Verification items for the finished model (mm, model axes). A direction names the side the tool comes from. Round coordinates to 2 decimals unless told otherwise and drop trailing zeros. Write each loop counter-clockwise with the first axis right and the second up, starting at its lowest first coordinate (ties: lowest second). Pieces come first, ordered by that corner, then holes. Notation, with made-up numbers: (-10, 3) - (25, 3) arc R20 cw to (25, 40) - close; hole circle Ø9 at (3.5, 35). An arc over 180 degrees is marked (long way). Answer as a JSON object with one key per item and string values.
```python
from build123d import *

# Parameters (mm, degrees)
SKIZZE1_W                       = 100
SKIZZE1_H                       = 66
AUFSATZ_LINEAR_AUSTRAGEN1_DEPTH = 1.5
SKIZZE2_W                       = 61
SKIZZE2_H                       = 14
AUFSATZ_LINEAR_AUSTRAGEN2_DEPTH = 14
SKIZZE6_W                       = 82.5
SKIZZE6_H                       = 14
AUFSATZ_LINEAR_AUSTRAGEN4_DEPTH = 4
SKIZZE3_R                       = 3
AUFSATZ_LINEAR_AUSTRAGEN3_DEPTH = 20
DURCHGANGSLOCH_F_R_M31_D        = 3.4
SKIZZE7_W                       = 35
SKIZZE7_H                       = 18
AUFSATZ_LINEAR_AUSTRAGEN5_DEPTH = 10


with BuildPart() as part:
    # Skizze1 → Aufsatz-Linear austragen1 (new body)
    with BuildSketch(Plane(origin=(0, 0, 0), x_dir=(1, 0, 0), z_dir=(0, 1, 0))):
        Rectangle(SKIZZE1_W, SKIZZE1_H)
    extrude(amount=AUFSATZ_LINEAR_AUSTRAGEN1_DEPTH)

    # Skizze2 → Aufsatz-Linear austragen2 (add)
    with BuildSketch(Plane(origin=(0, 1.5, 0), x_dir=(1, 0, 0), z_dir=(0, 1, 0))):
        with Locations((0.5, 21)):
            Rectangle(SKIZZE2_W, SKIZZE2_H)
    extrude(amount=AUFSATZ_LINEAR_AUSTRAGEN2_DEPTH)

    # Skizze6 → Aufsatz-Linear austragen4 (add)
    with BuildSketch(Plane(origin=(0, 1.5, 0), x_dir=(1, 0, 0), z_dir=(0, 1, 0))):
        with Locations((0.5, 21)):
            Rectangle(SKIZZE6_W, SKIZZE6_H)
    extrude(amount=AUFSATZ_LINEAR_AUSTRAGEN4_DEPTH)

    # Skizze3 → Aufsatz-Linear austragen3 (add)
    with BuildSketch(Plane(origin=(0, 1.5, 0), x_dir=(1, 0, 0), z_dir=(0, 1, 0))):
        with Locations((34, 1.5)):
            Circle(SKIZZE3_R)
    extrude(amount=AUFSATZ_LINEAR_AUSTRAGEN3_DEPTH)

    # Durchgangsloch für M31 (through all)
    with Locations(Plane(origin=(0, 1.5, 0), x_dir=(1, 0, 0), z_dir=(0, 1, 0))):
        with Locations((-46, -27.400776428), (-46, 27.400776428), (46, 27.400776428), (46, -27.400776428)):
            Hole(DURCHGANGSLOCH_F_R_M31_D / 2)

    # Skizze7 → Aufsatz-Linear austragen5 (add)
    with BuildSketch(Plane(origin=(0, 1.5, 0), x_dir=(1, 0, 0), z_dir=(0, 1, 0))):
        with Locations((-24.5, -0.5)):
            Rectangle(SKIZZE7_W, SKIZZE7_H)
    extrude(amount=AUFSATZ_LINEAR_AUSTRAGEN5_DEPTH)


solid = part.part
```
1. Material ranges on probe 1 along Z at (x, y) = (-46, 0.9); probe 2 along Z at (x, y) = (-20, 6); probe 3 along Y at (x, z) = (-39, 23), recorded low to high. Write a range as from..to.
Completed:
{"probe 1": "z = -33..-29.1, -25.7..25.7, 29.1..33", "probe 2": "z = -28..-14, -8.5..9.5", "probe 3": "y = 0..1.5"}
2. Go/stop test with flat-tipped pins: pin 1 (2 mm diameter, centred on x = 46, z = 27.4, fed in from +Y); pin 2 (10 mm diameter, centred on x = 14.5, z = -17, fed in from +Y); pin 3 (8.5 mm diameter, centred on x = 36.5, z = -21.5, fed in from +Y); pin 4 (1 mm diameter, centred on x = -5, y = 7, fed in from +Z). Record where each tip stops, or that it passes through.
Completed:
{"pin 1": "passes through", "pin 2": "stops at y = 15.5", "pin 3": "stops at y = 5.5", "pin 4": "stops at z = -14"}
3. Cross-section at B-B (y = 8.75). Record the boundary of the cut face in (x, z).
Completed:
{"outline": "(-42, -8.5) - (-7, -8.5) - (-7, 9.5) - (-42, 9.5) - close; (-30, -28) - (31, -28) - (31, -14) - (-30, -14) - close; circle Ø6 at (34, -1.5)"}
4. Cross-section at D-D (x = 15). Record the boundary of the cut face in (y, z).
Completed:
{"outline": "(0, -33) - (1.5, -33) - (1.5, -28) - (15.5, -28) - (15.5, -14) - (1.5, -14) - (1.5, 33) - (0, 33) - close"}
5. Cross-section at A-A (x = -46). Record the boundary of the cut face in (y, z), plus the area to 3 significant figures.
Completed:
{"outline": "(0, -33) - (1.5, -33) - (1.5, -29.1) - (0, -29.1) - close; (0, -25.7) - (1.5, -25.7) - (1.5, 25.7) - (0, 25.7) - close; (0, 29.1) - (1.5, 29.1) - (1.5, 33) - (0, 33) - close", "area": "88.8 mm^2"}
6. Access from +Z, -Z, +X, -X, +Y, -Y to the whole of each face (thin tool, end or side, straight path). Record for faces 4 (the face through (-42, 6, 1)), 5 (the face through (31, 11.4, -1.6)), 6 (the face through (0, 8, -28)), 7 (the face through (-25, 11.5, 0)).
Completed:
{"face 4": "+Z, -Z, -X, +Y", "face 5": "+Y", "face 6": "-Z, +X, -X, +Y", "face 7": "+Z, -X, +Y"}
7. Mould release check, pull along Z, two halves, no side actions. Record for faces 1 (the face through (36, 5.5, -21)), 2 (the face through (-25, 6, -8.5)), 3 (the face through (-25, 6, 9.5)): released by +Z, released by -Z, zero draft, split by the parting line, or undercut.
Completed:
{"face 1": "zero draft", "face 2": "undercut", "face 3": "released by +Z"}
8. Cross-section at C-C (z = -22.5). Record the boundary of the cut face in (x, y), plus the area to 3 significant figures.
Completed:
{"outline": "(-50, 0) - (50, 0) - (50, 1.5) - (41.75, 1.5) - (41.75, 5.5) - (31, 5.5) - (31, 15.5) - (-30, 15.5) - (-30, 5.5) - (-40.75, 5.5) - (-40.75, 1.5) - (-50, 1.5) - close", "area": "1,090 mm^2"}
